from build123d import *

# Parameters (mm, degrees)
SKETCH1_W           = 80
SKETCH1_H           = 130
BOSS_EXTRUDE1_DEPTH = 3
SKETCH2_W           = 80
SKETCH2_H           = 2
BOSS_EXTRUDE2_DEPTH = 80
FILLET1_DEPTH       = 80
CUT_EXTRUDE1_DEPTH  = 174.749820144
CUT_EXTRUDE2_START  = -3
CUT_EXTRUDE2_DEPTH  = 171.749820238
CHAMFER1_SIZE2      = 28.543093363
CHAMFER1_SIZE       = 3
CHAMFER2_SIZE       = 30


with BuildPart() as part:
    # Sketch1 → Boss-Extrude1 (new body)
    with BuildSketch(Plane(origin=(0, 0, 0), x_dir=(1, 0, 0), z_dir=(0, 1, 0))):
        with Locations((40, 65)):
            Rectangle(SKETCH1_W, SKETCH1_H)
    extrude(amount=BOSS_EXTRUDE1_DEPTH)

    # Sketch2 → Boss-Extrude2 (add)
    with BuildSketch(Plane(origin=(0, 3, 0), x_dir=(1, 0, 0), z_dir=(0, 1, 0))):
        with Locations((40, 129)):
            Rectangle(SKETCH2_W, SKETCH2_H)
    extrude(amount=BOSS_EXTRUDE2_DEPTH)

    # Fillet1: read off the stored shape, not the designer's step
    # Fillet1 outline → Fillet1 (add)
    with BuildSketch(Plane.YZ):
        with BuildLine():
            Line((3, -128), (83, -128))
            ThreePointArc((83, -128), (26.431457505, -104.568542495), (3, -48))
            Line((3, -48), (3, -128))
        make_face()
    extrude(amount=FILLET1_DEPTH)

    # Sketch3 → Cut-Extrude1 (cut, through all)
    with BuildSketch(Plane(origin=(0, 0, -130), x_dir=(-1, 0, 0), z_dir=(0, 0, -1))):
        with BuildLine():
            Line((-38.4, 73), (-38.4, 36.5))
            ThreePointArc((-38.4, 36.5), (-40, 34.9), (-41.6, 36.5))
            Line((-41.6, 36.5), (-41.6, 73))
            ThreePointArc((-41.6, 73), (-40, 74.6), (-38.4, 73))
        make_face()
        with BuildLine():
            Line((-53.4, 73), (-53.4, 36.5))
            ThreePointArc((-53.4, 36.5), (-55, 34.9), (-56.6, 36.5))
            Line((-56.6, 36.5), (-56.6, 73))
            ThreePointArc((-56.6, 73), (-55, 74.6), (-53.4, 73))
        make_face()
        with BuildLine():
            Line((-71.6, 36.5), (-71.6, 73))
            ThreePointArc((-71.6, 73), (-70, 74.6), (-68.4, 73))
            Line((-68.4, 73), (-68.4, 36.5))
            ThreePointArc((-68.4, 36.5), (-70, 34.9), (-71.6, 36.5))
        make_face()
        with BuildLine():
            Line((-23.4, 73), (-23.4, 36.5))
            ThreePointArc((-23.4, 36.5), (-25, 34.9), (-26.6, 36.5))
            Line((-26.6, 36.5), (-26.6, 73))
            ThreePointArc((-26.6, 73), (-25, 74.6), (-23.4, 73))
        make_face()
        with BuildLine():
            Line((-11.6, 36.5), (-11.6, 73))
            ThreePointArc((-11.6, 73), (-10, 74.6), (-8.4, 73))
            Line((-8.4, 73), (-8.4, 36.5))
            ThreePointArc((-8.4, 36.5), (-10, 34.9), (-11.6, 36.5))
        make_face()
    extrude(amount=-CUT_EXTRUDE1_DEPTH, mode=Mode.SUBTRACT)

    # Sketch4 → Cut-Extrude2 (cut, through all)
    with BuildSketch(Plane(origin=(0, 0, -130), x_dir=(-1, 0, 0), z_dir=(0, 0, -1)).offset(CUT_EXTRUDE2_START)):
        with BuildLine():
            Line((-66.4, 73), (-66.4, 36.5))
            ThreePointArc((-66.4, 36.5), (-70, 32.9), (-73.6, 36.5))
            Line((-73.6, 36.5), (-73.6, 73))
            ThreePointArc((-73.6, 73), (-70, 76.6), (-66.4, 73))
        make_face()
        with BuildLine():
            Line((-51.4, 73), (-51.4, 36.5))
            ThreePointArc((-51.4, 36.5), (-55, 32.9), (-58.6, 36.5))
            Line((-58.6, 36.5), (-58.6, 73))
            ThreePointArc((-58.6, 73), (-55, 76.6), (-51.4, 73))
        make_face()
        with BuildLine():
            Line((-43.6, 36.5), (-43.6, 73))
            ThreePointArc((-43.6, 73), (-40, 76.6), (-36.4, 73))
            Line((-36.4, 73), (-36.4, 36.5))
            ThreePointArc((-36.4, 36.5), (-40, 32.9), (-43.6, 36.5))
        make_face()
        with BuildLine():
            Line((-21.4, 73), (-21.4, 36.5))
            ThreePointArc((-21.4, 36.5), (-25, 32.9), (-28.6, 36.5))
            Line((-28.6, 36.5), (-28.6, 73))
            ThreePointArc((-28.6, 73), (-25, 76.6), (-21.4, 73))
        make_face()
        with BuildLine():
            Line((-13.6, 36.5), (-13.6, 73))
            ThreePointArc((-13.6, 73), (-10, 76.6), (-6.4, 73))
            Line((-6.4, 73), (-6.4, 36.5))
            ThreePointArc((-6.4, 36.5), (-10, 32.9), (-13.6, 36.5))
        make_face()
    extrude(amount=-CUT_EXTRUDE2_DEPTH, mode=Mode.SUBTRACT)

    # Chamfer1
    chamfer1_edges = [part.edges().sort_by_distance(p)[0] for p in [
        (40, 3, 0),
    ]]
    chamfer1_side = [part.faces().sort_by_distance(p)[0] for p in [
        (40, 2.94, 0),
    ]]
    chamfer(chamfer1_edges, length=CHAMFER1_SIZE - 0.0001, length2=CHAMFER1_SIZE2 - 0.0001, reference=chamfer1_side[0])  # a hair under: the kernel refuses the full size

    # Chamfer2
    chamfer2_edges = [part.edges().sort_by_distance(p)[0] for p in [
        (40, 0, -130),
    ]]
    chamfer(chamfer2_edges, length=CHAMFER2_SIZE)


solid = part.part
Verification items for the finished model (mm, model axes). A direction names the side the tool comes from. Round coordinates to 2 decimals unless told otherwise and drop trailing zeros. Loops run counter-clockwise (first coordinate to the right, second up) from the corner with the lowest first, then second, coordinate; pieces in that order, holes last. Notation, with made-up numbers: (-7, 85) - (25, 85) arc R29 cw to (25, 116) - close; hole circle Ø5 at (27.5, 9.5). An arc over 180 degrees is marked (long way). Use a Markdown table: item, result. Add a question column.
1. Thickness scan on probe 1 along Y at (x, z) = (35, -44.5); probe 2 along Z at (x, y) = (28, 49.5); probe 3 along Y at (x, z) = (25, -55.5). Record the ranges inside material, lowest first. Write a range as [from, to].
2. Section check D-D, the plane y = 40.5. Give the number of separate pieces and of enclosed holes in the cut face, plus the area to 3 significant figures.
3. Section check B-B, the plane z = -115. Record the boundary of the cut face in (x, y), plus the area to 3 significant figures.
4. Access from +Z, -Z, +X, -X, +Y, -Y to the whole of each face (thin tool, end or side, straight path). Record for faces 4 (the face through (26.6, 54, -129)), 5 (the face through (24.9, 32.9, -118.8)), 6 (the face through (0, 20, -103)).
5. Gauge pin test, flat ends, axial feed: pin 1 (6 mm diameter, centred on x = 26.5, y = 55, fed in from +Z); pin 2 (21.5 mm diameter, centred on x = 45.5, z = -39, fed in from +Y); pin 3 (8 mm diameter, centred on x = 48.5, z = -114, fed in from +Y). Record the tip position at first contact, or that the pin passes through.
6. Release check for a two-part mould opening along Y. For faces 1 (the face through (39.44, 1.52, -14.47)), 2 (the face through (58.6, 46, -123)), 3 (the face through (55, 34.9, -128.5)) record: released by +Y, released by -Y, zero draft, split by the parting line, or undercut.
Checks:
| question | item | result |
|---|---|---|
| 1 | probe 1 | y = [0, 3] |
| 1 | probe 2 | z = [-130, -127] |
| 1 | probe 3 | y = [0, 3.35] |
| 2 | separate pieces | 6 |
| 2 | enclosed holes | 0 |
| 2 | area | 686 mm^2 |
| 3 | outline | (0, 15) - (80, 15) - (80, 39.29) - (73.6, 39.29) - (73.6, 36.5) arc R3.6 cw to (66.4, 36.5) - (66.4, 39.29) - (58.6, 39.29) - (58.6, 36.5) arc R3.6 cw to (51.4, 36.5) - (51.4, 39.29) - (43.6, 39.29) - (43.6, 36.5) arc R3.6 cw to (36.4, 36.5) - (36.4, 39.29) - (28.6, 39.29) - (28.6, 36.5) arc R3.6 cw to (21.4, 36.5) - (21.4, 39.29) - (13.6, 39.29) - (13.6, 36.5) arc R3.6 cw to (6.4, 36.5) - (6.4, 39.29) - (0, 39.29) - close |
| 3 | area | 1,740 mm^2 |
| 4 | face 4 | +Z, -Z |
| 4 | face 5 | +Z, +Y |
| 4 | face 6 | +Z, -Z, -X, +Y, -Y |
| 5 | pin 1 | stops at z = -122.1 |
| 5 | pin 2 | stops at y = 3.02 |
| 5 | pin 3 | stops at y = 44.27 |
| 6 | face 1 | released by +Y |
| 6 | face 2 | zero draft |
| 6 | face 3 | undercut |
